The model under review builds one solid part; all positions refer to its coordinate system, in mm. Round coordinates to 2 decimals unless told otherwise and drop trailing zeros. Loops run counter-clockwise (first coordinate to the right, second up) from the corner with the lowest first, then second, coordinate; pieces in that order, holes last. Notation, with made-up numbers: M -36,30.5 L 13,30.5 A33 cw 13,62.5 Z; hole C 52.25,51 d3. An arc over 180 degrees is marked long. One line per question, with ' | ' between items.
from build123d import *

# Parameters (mm, degrees)
MODEL_R                 = 1.5
SALIENTE_EXTRUIR1_DEPTH = 3


with BuildPart() as part:
    # Model → Saliente-Extruir1 (new body)
    with BuildSketch(Plane.XY):
        with BuildLine():
            Line((-105.943383637, 101.056539338), (-105.943383637, 74.056539338))
            ThreePointArc((-105.943383637, 74.056539338), (-104.625364152, 70.874558823), (-101.443383637, 69.556539338))
            Line((-101.443383637, 69.556539338), (-74.443383637, 69.556539338))
            ThreePointArc((-74.443383637, 69.556539338), (-71.261403122, 70.874558823), (-69.943383637, 74.056539338))
            Line((-69.943383637, 74.056539338), (-69.943383637, 101.056539338))
            ThreePointArc((-69.943383637, 101.056539338), (-71.261403122, 104.238519853), (-74.443383637, 105.556539338))
            Line((-74.443383637, 105.556539338), (-101.443383637, 105.556539338))
            ThreePointArc((-101.443383637, 105.556539338), (-104.625364152, 104.238519853), (-105.943383637, 101.056539338))
        make_face()
        with Locations((-101.443383637, 101.056539338)):
            Circle(MODEL_R, mode=Mode.SUBTRACT)
        with Locations((-92.443383637, 101.056539338)):
            Circle(MODEL_R, mode=Mode.SUBTRACT)
        with Locations((-83.443383637, 101.056539338)):
            Circle(MODEL_R, mode=Mode.SUBTRACT)
        with Locations((-74.443383637, 101.056539338)):
            Circle(MODEL_R, mode=Mode.SUBTRACT)
        with Locations((-101.443383637, 92.056539338)):
            Circle(MODEL_R, mode=Mode.SUBTRACT)
        with Locations((-92.443383637, 92.056539338)):
            Circle(MODEL_R, mode=Mode.SUBTRACT)
        with Locations((-83.443383637, 92.056539338)):
            Circle(MODEL_R, mode=Mode.SUBTRACT)
        with Locations((-74.443383637, 92.056539338)):
            Circle(MODEL_R, mode=Mode.SUBTRACT)
        with Locations((-101.443383637, 83.056539338)):
            Circle(MODEL_R, mode=Mode.SUBTRACT)
        with Locations((-92.443383637, 83.056539338)):
            Circle(MODEL_R, mode=Mode.SUBTRACT)
        with Locations((-83.443383637, 83.056539338)):
            Circle(MODEL_R, mode=Mode.SUBTRACT)
        with Locations((-74.443383637, 83.056539338)):
            Circle(MODEL_R, mode=Mode.SUBTRACT)
        with Locations((-101.443383637, 74.056539338)):
            Circle(MODEL_R, mode=Mode.SUBTRACT)
        with Locations((-92.443383637, 74.056539338)):
            Circle(MODEL_R, mode=Mode.SUBTRACT)
        with Locations((-83.443383637, 74.056539338)):
            Circle(MODEL_R, mode=Mode.SUBTRACT)
        with Locations((-74.443383637, 74.056539338)):
            Circle(MODEL_R, mode=Mode.SUBTRACT)
    extrude(amount=SALIENTE_EXTRUIR1_DEPTH)


solid = part.part
1) Add section A-A on y = 93. State the section outline as (x, z) points, then the cut area to 3 significant figures.
Output values:
outline: M -105.94,0 L -102.61,0 L -102.61,3 L -105.94,3 Z; M -100.28,0 L -93.61,0 L -93.61,3 L -100.28,3 Z; M -91.28,0 L -84.61,0 L -84.61,3 L -91.28,3 Z; M -82.28,0 L -75.61,0 L -75.61,3 L -82.28,3 Z; M -73.28,0 L -69.94,0 L -69.94,3 L -73.28,3 Z | area: 80.0 mm²
2) Add section B-B on x = -101. State the section outline as (y, z) points.
Output values:
outline: M 69.56,0 L 72.62,0 L 72.62,3 L 69.56,3 Z; M 75.49,0 L 81.62,0 L 81.62,3 L 75.49,3 Z; M 84.49,0 L 90.62,0 L 90.62,3 L 84.49,3 Z; M 93.49,0 L 99.62,0 L 99.62,3 L 93.49,3 Z; M 102.49,0 L 105.56,0 L 105.56,3 L 102.49,3 Z
3) Mouldability with a two-part tool opening along X and no side actions: class faces 1 (the cylindrical face through (-71.227, 104.203, 1.479)), 2 (the flat face through (-88, 105.557, 1)), 3 (the cylindrical face through (-100.013, 74.507, 1.479)), 4 (the cylindrical face through (-104.66, 70.91, 1.48)) as +X half, -X half, draft (parallel to the pull), parting line (faces both ways), or undercut.
Output values:
face 1: +X half | face 2: draft | face 3: undercut | face 4: -X half
4) For line 1 (X direction, y = 73, z = 0.5); line 2 (Y direction, x = -91.5, z = 2.5); line 3 (X direction, y = 101.5, z = 1), list the stretches that pass through material, from the lowest coordinate up.
Output values:
line 1: x = -105.82 to -102.51, -100.38 to -93.51, -91.38 to -84.51, -82.38 to -75.51, -73.38 to -70.07 | line 2: y = 69.56 to 72.89, 75.22 to 81.89, 84.22 to 90.89, 93.22 to 99.89, 102.22 to 105.56 | line 3: x = -105.92 to -102.88, -100.01 to -93.88, -91.01 to -84.88, -82.01 to -75.88, -73.01 to -69.97
5) Add section C-C on z = 2.55. State how many separate pieces and enclosed holes the cut face has, then the cut area to 3 significant figures.
Output values:
separate pieces: 1 | enclosed holes: 16 | area: 1,170 mm²
6) Insertion check: P1, Ø2.5, axis at x = -74.44, y = 101.06, coming from the -Z side. The pin has a flat end and moves straight along its axis. Give the tip position at first contact, or say it passes through.
Output values:
P1: passes through
